Could you check a few things on this drawing? It's one solid part, dimensions in mm from its lowest x, y, z. A direction names the side the tool comes from. Coordinates: 2 decimals unless noted, no trailing zeros. Write each loop counter-clockwise with the first axis right and the second up, starting at its lowest first coordinate (ties: lowest second). Pieces come first, ordered by that corner, then holes. Notation, with made-up numbers: (-20, 58) - (18, 58) arc R27 cw to (18, 81) - close; hole circle Ø4 at (-30, -40). An arc over 180 degrees is marked (long way). Answer as a JSON object with one key per item and string values. Group by question number.
1) If we section it at A-A (x = 2.5): Write out the boundary of the cut face in (y, z).
2) Will these pins go through, and if not, where does the flat tip stop? pin 1 Ø0.9 at (x, z) = (2, 8.5) entering from -Y; pin 2 Ø0.9 at (x, z) = (2, 15.5) entering from +Y.
3) On a 3-axis mill with a long thin cutter (end or side, diameter ignored), from which of +Z, -Z, +X, -X, +Y, -Y can I reach the whole of each face in a straight line? I mean the marked faces 1, 2 and 3. Say none if no direction works.
4) Please list where these lines run through material, in increasing order: line 1 along Z through (x, y) = (2.65, 14); line 2 along X through (y, z) = (64, 12); line 3 along Y through (x, z) = (3.8, 10.5).
5) If we section it at C-C (y = 70): Write out the boundary of the cut face in (x, z), plus the area to 3 significant figures.
6) If we section it at D-D (y = 34.5): Write out the boundary of the cut face in (x, z).
7) If we section it at B-B (z = 20.5): Write out the boundary of the cut face in (x, y), plus the area to 3 significant figures.
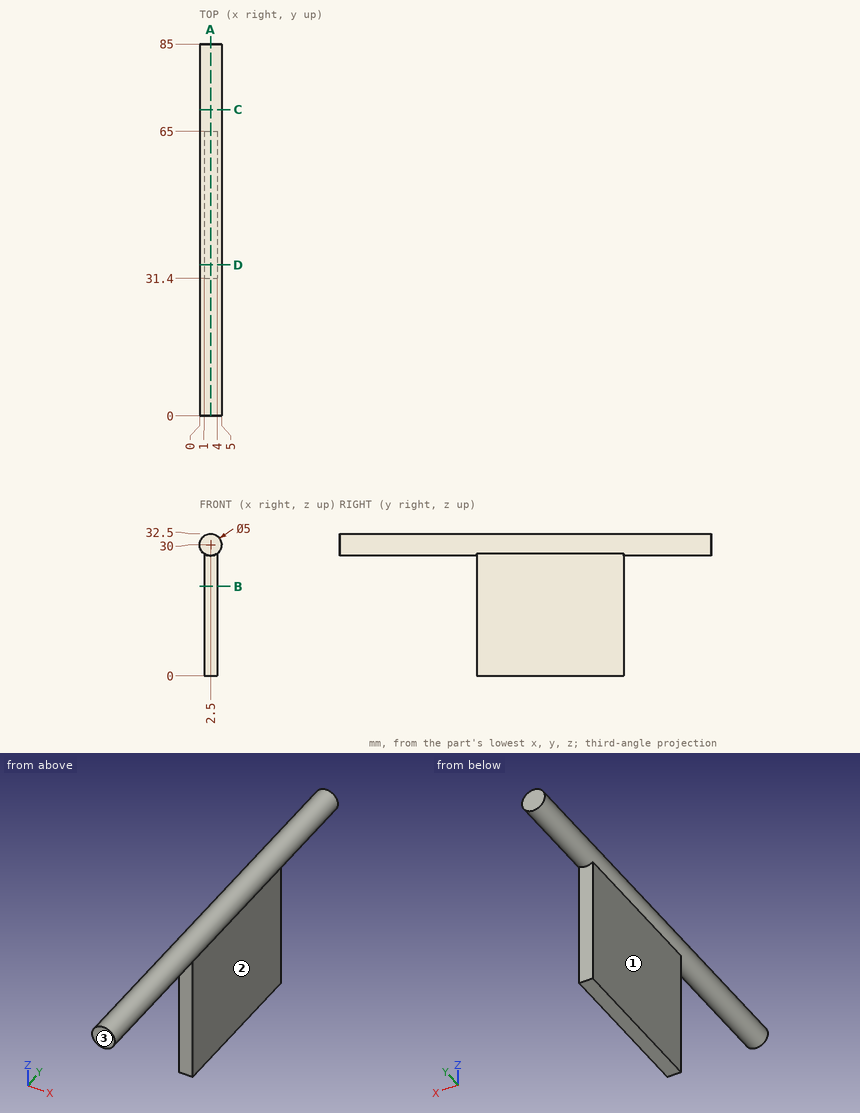
Here are the results:
{
 "1": {"outline": "(0, 27.5) - (31.4, 27.5) - (31.4, 0) - (65, 0) - (65, 27.5) - (85, 27.5) - (85, 32.5) - (0, 32.5) - close"},
 "2": {"pin 1": "stops at y = 31.4", "pin 2": "stops at y = 65"},
 "3": {"face 1": "-Z, -X, +Y, -Y", "face 2": "-Z, +X, +Y, -Y", "face 3": "+Z, -Z, +X, -X, -Y"},
 "4": {"line 1": "z = 27.5 to 32.5", "line 2": "x = 1 to 4", "line 3": "y = 31.4 to 65"},
 "5": {"outline": "circle Ø5 at (2.5, 30)", "area": "19.6 mm²"},
 "6": {"outline": "(1, 0) - (4, 0) - (4, 28) arc R2.5 ccw (long way) to (1, 28) - close"},
 "7": {"outline": "(1, 31.4) - (4, 31.4) - (4, 65) - (1, 65) - close", "area": "101 mm²"}
}
